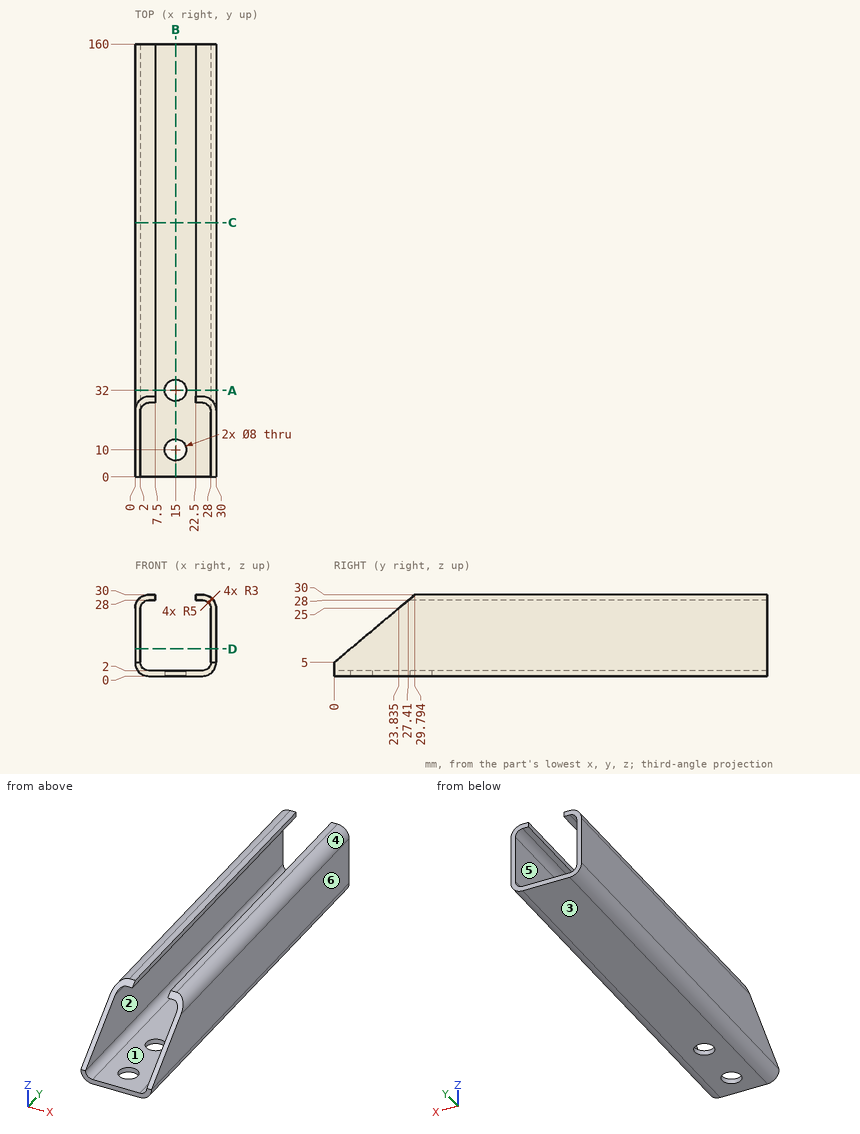
Check sheet for the drawn part. Datum: minimum x, y, z corner. Units: mm. A direction names the side the tool comes from. Round coordinates to 2 decimals unless told otherwise and drop trailing zeros. Order: outer loops, then holes, each group sorted by start corner. A loop starts at its lowest first (then second) coordinate and runs counter-clockwise, first axis right, second up.
(1) Cross-section at B-B, the plane x = 15. Enter the section's corners in (y, z).
(2) Cross-section at D-D, the plane z = 10. Enter the section's corners in (x, y).
(3) Go/stop test with flat-tipped pins: P1, Ø3, axis at x = 26, z = 3.5, coming from the -Y side; P2, Ø1, axis at x = 15, y = 57.5, coming from the +Z side; P3, Ø7, axis at x = 15, y = 10, coming from the -Z side; P4, Ø0.6, axis at y = 72.5, z = 29, coming from the -X side. Record where each tip stops, or that it passes through.
(4) Scan lines: probe 1 along Y at (x, z) = (15, 1.4); probe 2 along X at (y, z) = (83, 19.5); probe 3 along X at (y, z) = (10, 1). Record each from-to range of solid material in increasing order.
(5) Cross-section at A-A, the plane y = 32. Enter the section's corners in (x, z).
(6) Draft check along Z on the marked faces 1, 2, 3 and 4. Enter one of: pulls with the +Z half, pulls with the -Z half, needs draft (parallel to the pull), parting line crosses it, or undercut.
(7) Access from +Z, -Z, +X, -X, +Y, -Y to the whole of each face (thin tool, end or side, straight path). Record for the marked faces 5 and 6.
(8) Cross-section at C-C, the plane y = 94. Enter the section's corners in (x, z).
Check sheet entries:
1. outline: (0, 0) - (6, 0) - (6, 2) - (0, 2) - close; (14, 0) - (28, 0) - (28, 2) - (14, 2) - close; (36, 0) - (160, 0) - (160, 2) - (36, 2) - close
2. outline: (0, 5.96) - (2, 5.96) - (2, 160) - (0, 160) - close; (28, 5.96) - (30, 5.96) - (30, 160) - (28, 160) - close
3. P1: stops at y = 0
3. P2: stops at z = 2
3. P3: passes through
3. P4: stops at x = 1.64
4. probe 1: y = 0 to 6, 14 to 28, 36 to 160
4. probe 2: x = 0 to 2, 28 to 30
4. probe 3: x = 2 to 11, 19 to 28
5. outline: (0, 5) arc R5 ccw to (5, 0) - (11, 0) - (11, 2) - (5, 2) arc R3 cw to (2, 5) - (2, 25) arc R3 cw to (5, 28) - (7.5, 28) - (7.5, 30) - (5, 30) arc R5 ccw to (0, 25) - close; (19, 0) - (25, 0) arc R5 ccw to (30, 5) - (30, 25) arc R5 ccw to (25, 30) - (22.5, 30) - (22.5, 28) - (25, 28) arc R3 cw to (28, 25) - (28, 5) arc R3 cw to (25, 2) - (19, 2) - close
6. face 1: undercut
6. face 2: undercut
6. face 3: pulls with the -Z half
6. face 4: pulls with the +Z half
7. face 5: +Y, -Y
7. face 6: +Z, -Z, +X, +Y, -Y
8. outline: (0, 5) arc R5 ccw to (5, 0) - (25, 0) arc R5 ccw to (30, 5) - (30, 25) arc R5 ccw to (25, 30) - (22.5, 30) - (22.5, 28) - (25, 28) arc R3 cw to (28, 25) - (28, 5) arc R3 cw to (25, 2) - (5, 2) arc R3 cw to (2, 5) - (2, 25) arc R3 cw to (5, 28) - (7.5, 28) - (7.5, 30) - (5, 30) arc R5 ccw to (0, 25) - close
